Input: part model. Units: mm. Frame: model coordinates. A direction names the side the tool comes from. Give positions to 0.01 mm unless a question says otherwise; leave off trailing zeros. Loops run counter-clockwise (first coordinate to the right, second up) from the corner with the lowest first, then second, coordinate; pieces in that order, holes last.
from build123d import *

# Parameters (mm, degrees)
CROQUIS1_W              = 10
CROQUIS1_H              = 25
SALIENTE_EXTRUIR1_DEPTH = 28
CROQUIS2_R              = 12.5
SALIENTE_EXTRUIR2_DEPTH = 12
REDONDEO1_R             = 5
CORTAR_EXTRUIR1_DEPTH   = 13
CROQUIS5_R              = 9.915
CORTAR_EXTRUIR2_DEPTH   = 7
CROQUIS8_R              = 1.175
CORTAR_EXTRUIR5_DEPTH   = 50.08411164
CROQUIS10_W             = 7
CROQUIS10_H             = 15
SALIENTE_EXTRUIR3_DEPTH = 5
CORTAR_EXTRUIR6_DEPTH   = 7
CORTAR_EXTRUIR7_DEPTH   = 3.85
CHAFL_N1_SIZE           = 4.3
CHAFL_N1_SIZE2          = 5.124540448
REDONDEO2_R             = 1
CORTAR_EXTRUIR8_DEPTH   = 4
REDONDEO3_R             = 3
CROQUIS14_R             = 12.5
CROQUIS14_R_2           = 11.25
SALIENTE_EXTRUIR4_DEPTH = 7.35
CROQUIS15_R             = 12.5
CROQUIS15_R_2           = 11
SALIENTE_EXTRUIR5_DEPTH = 1
CHAFL_N2_SIZE           = 0.5
CHAFL_N3_SIZE           = 0.5
CROQUIS16_R             = 6.5
CORTAR_EXTRUIR9_DEPTH   = 50.43149313


# Some blends are built 0.0001 mm under size
with BuildPart() as part:
    # Croquis1 → Saliente-Extruir1 (new body)
    with BuildSketch(Plane(origin=(0, 0, 0), x_dir=(1, 0, 0), z_dir=(0, 1, 0))):
        with Locations((-5, 12.5)):
            Rectangle(CROQUIS1_W, CROQUIS1_H)
    extrude(amount=SALIENTE_EXTRUIR1_DEPTH)

    # Croquis2 → Saliente-Extruir2 (add)
    with BuildSketch(Plane(origin=(0, 0, 0), x_dir=(0, 0, -1), z_dir=(1, 0, 0))):
        with Locations((12.5, 28)):
            Circle(CROQUIS2_R)
    extrude(amount=-SALIENTE_EXTRUIR2_DEPTH)

    # Croquis3 → Cortar-Revolución1 (revolve, cut)
    with BuildSketch(Plane(origin=(0, 0, 0), x_dir=(0, 0, -1), z_dir=(1, 0, 0))):
        Polygon((21, 0.5), (21, 4), (19, 4), (19, 10), (21, 10), (21, 15), (15.5, 15), (15.5, 41), (12.5, 41), (12.5, 0), (21, 0), align=None)
    revolve(axis=Axis((0, 0, -12.5), (0, 1, 0)), mode=Mode.SUBTRACT)

    # Redondeo1
    redondeo1_edges = [part.edges().sort_by_distance(p)[0] for p in [
        (-5, 0, -25),
        (-5, 0, 0),
    ]]
    fillet(redondeo1_edges, radius=REDONDEO1_R)

    # Croquis4 → Cortar-Extruir1 (cut)
    with BuildSketch(Plane.XZ.offset(-15)):
        Polygon((0, -18.67764788), (5.35, -15.58882394), (5.35, -9.41117606), (0, -6.32235212), (-5.35, -9.41117606), (-5.35, -15.58882394), align=None)
    extrude(amount=-CORTAR_EXTRUIR1_DEPTH, mode=Mode.SUBTRACT)

    # Croquis5 → Cortar-Extruir2 (cut)
    with BuildSketch(Plane(origin=(0, 0, 0), x_dir=(0, 0, -1), z_dir=(1, 0, 0))):
        with Locations((12.5, 28)):
            Circle(CROQUIS5_R)
    extrude(amount=-CORTAR_EXTRUIR2_DEPTH, mode=Mode.SUBTRACT)

    # Croquis8 → Cortar-Extruir5 (cut, through all)
    with BuildSketch(Plane(origin=(0, 0, 0), x_dir=(0, 0, -1), z_dir=(1, 0, 0))):
        with Locations((21.5, 16.5)):
            Circle(CROQUIS8_R)
        with Locations((3.5, 16.5)):
            Circle(CROQUIS8_R)
        with Locations((3.5, 7.5)):
            Circle(CROQUIS8_R)
        with Locations((21.5, 7.5)):
            Circle(CROQUIS8_R)
    extrude(amount=-CORTAR_EXTRUIR5_DEPTH, mode=Mode.SUBTRACT)

    # Croquis10 → Saliente-Extruir3 (add, symmetric)
    with BuildSketch(Plane.XY.offset(-12.5)):
        with Locations((-13.5, 0.5)):
            Rectangle(CROQUIS10_W, CROQUIS10_H)
    extrude(amount=SALIENTE_EXTRUIR3_DEPTH, both=True)

    # Croquis11 → Cortar-Extruir6 (cut)
    with BuildSketch(Plane.XZ.offset(7)):
        with BuildLine():
            Line((-10.743486399, -17.5), (-10, -17.5))
            Line((-10, -17.5), (-10, -7.5))
            Line((-10, -7.5), (-10.743486399, -7.5))
            ThreePointArc((-10.743486399, -7.5), (-11.85, -12.5), (-10.743486399, -17.5))
        make_face()
    extrude(amount=-CORTAR_EXTRUIR6_DEPTH, mode=Mode.SUBTRACT)

    # Croquis12 → Cortar-Extruir7 (cut)
    with BuildSketch(Plane.XZ.offset(7)):
        with BuildLine():
            Line((-13.787722048, -17.5), (-10.743486399, -17.5))
            ThreePointArc((-10.743486399, -17.5), (-11.85, -12.5), (-10.743486399, -7.5))
            Line((-10.743486399, -7.5), (-11.837335004, -7.5))
            ThreePointArc((-11.837335004, -7.5), (-12.358868803, -8.981355103), (-12.6958, -10.515267686))
            Line((-12.6958, -10.515267686), (-13.787722048, -17.5))
        make_face()
    extrude(amount=-CORTAR_EXTRUIR7_DEPTH, mode=Mode.SUBTRACT)

    # Chaflán1
    chafl_n1_edges = [part.edges().sort_by_distance(p)[0] for p in [
        (-17, 8, -12.5),
    ]]
    chafl_n1_side = [part.faces().sort_by_distance(p)[0] for p in [
        (-13.5, 8, -12.5),
    ]]
    chamfer(chafl_n1_edges, length=CHAFL_N1_SIZE, length2=CHAFL_N1_SIZE2, reference=chafl_n1_side[0])

    # Redondeo2
    redondeo2_edges = [part.edges().sort_by_distance(p)[0] for p in [
        (-12.358868803, -3.15, -8.981355103),
        (-13.241761024, -3.15, -14.007633843),
    ]]
    fillet(redondeo2_edges, radius=REDONDEO2_R - 0.0001)  # a hair under: the kernel refuses the full size

    # Croquis13 → Cortar-Extruir8 (cut)
    with BuildSketch(Plane.ZY.offset(10)):
        Polygon((-21.5, 18.830940108), (-23.518653348, 17.665470054), (-23.518653348, 15.334529946), (-21.5, 14.169059892), (-19.481346652, 15.334529946), (-19.481346652, 17.665470054), align=None)
        Polygon((-3.5, 18.830940108), (-5.518653348, 17.665470054), (-5.518653348, 15.334529946), (-3.5, 14.169059892), (-1.481346652, 15.334529946), (-1.481346652, 17.665470054), align=None)
        Polygon((-3.5, 9.830940108), (-5.518653348, 8.665470054), (-5.518653348, 6.334529946), (-3.5, 5.169059892), (-1.481346652, 6.334529946), (-1.481346652, 8.665470054), align=None)
        Polygon((-21.5, 9.830940108), (-23.518653348, 8.665470054), (-23.518653348, 6.334529946), (-21.5, 5.169059892), (-19.481346652, 6.334529946), (-19.481346652, 8.665470054), align=None)
    extrude(amount=-CORTAR_EXTRUIR8_DEPTH, mode=Mode.SUBTRACT)

    # Redondeo3
    redondeo3_edges = [part.edges().sort_by_distance(p)[0] for p in [
        (-17, 2.875459552, -12.5),
        (-12.7, 8, -12.5),
    ]]
    fillet(redondeo3_edges, radius=REDONDEO3_R)

    # Croquis14 → Saliente-Extruir4 (add)
    with BuildSketch(Plane.ZY.offset(12)):
        with Locations((-12.5, 28)):
            Circle(CROQUIS14_R)
        with Locations((-12.5, 28)):
            Circle(CROQUIS14_R_2, mode=Mode.SUBTRACT)
    extrude(amount=SALIENTE_EXTRUIR4_DEPTH)

    # Croquis15 → Saliente-Extruir5 (add)
    with BuildSketch(Plane.ZY.offset(19.35)):
        with Locations((-12.5, 28)):
            Circle(CROQUIS15_R)
        with Locations((-12.5, 28)):
            Circle(CROQUIS15_R_2, mode=Mode.SUBTRACT)
    extrude(amount=SALIENTE_EXTRUIR5_DEPTH)

    # Chaflán2
    chafl_n2_edges = [part.edges().sort_by_distance(p)[0] for p in [
        (-20.35, 28, -23.5),
    ]]
    chamfer(chafl_n2_edges, length=CHAFL_N2_SIZE)

    # Chaflán3
    # the kernel refuses this chamfer: 0.5 mm, written as the material it takes off along each edge
    with BuildSketch(Plane(origin=(-19.35, 28, -12.5), x_dir=(0, 0, 1), z_dir=(0, -1, 0))) as chafl_n3_piece_1_section:
        Polygon((11, CHAFL_N3_SIZE), (11 + CHAFL_N3_SIZE, 0), (11, 0), align=None)
    chafl_n3_piece_1 = revolve(axis=Axis((-19.35, 28, -12.5), (-1, 0, 0)), mode=Mode.PRIVATE)
    chafl_n3_piece_1 = chafl_n3_piece_1 & Plane(origin=(-19.718458847, 28, -12.5), x_dir=(0, 0, 1), z_dir=(1, 0, 0)) * Cylinder(11.25, 46, mode=Mode.PRIVATE)
    add(chafl_n3_piece_1, mode=Mode.SUBTRACT)

    # Croquis16 → Cortar-Extruir9 (cut, through all)
    with BuildSketch(Plane(origin=(-7, 0, 0), x_dir=(0, 0, -1), z_dir=(1, 0, 0))):
        with Locations((12.5, 28)):
            Circle(CROQUIS16_R)
    extrude(amount=-CORTAR_EXTRUIR9_DEPTH, mode=Mode.SUBTRACT)


solid = part.part
(1) Ray query, probe 1 along Z at (x, y) = (-6.25, 17); probe 2 along Y at (x, z) = (-19.5, -12.5); probe 3 along Y at (x, z) = (-9.25, -1.75). Return the intervals inside material, ascending.
Values follow:
probe 1: z = -25 to -23.52, -19.48 to -5.52, -1.48 to 0
probe 2: y = 15.5 to 16.75, 39.25 to 40.5
probe 3: y = 1.2 to 6.18, 8.82 to 15.18, 17.82 to 34.38
(2) Pin query (flat end, axial travel): pin 1 Ø1.2 at (y, z) = (6.5, -21) entering from -X; pin 2 Ø1.5 at (y, z) = (11, -8.5) entering from -X; pin 3 Ø2 at (y, z) = (31, -9) entering from -X; pin 4 Ø1.5 at (x, z) = (-5.5, -3) entering from -Y. Return the tip coordinate at first contact, or that it passes through.
Values follow:
pin 1: stops at x = -6
pin 2: stops at x = -10
pin 3: passes through
pin 4: stops at y = 0.16
(3) Cut plane B-B (y = 7.5). Return the cut outline in (x, z) (3 decimals).
Values follow:
outline: (-12.959, -17.5) - (-10, -17.5) - (-10, -19.481) - (-6, -19.481) - (-6, -20.325) - (0, -20.325) - (0, -19) arc R6.5 cw to (0, -6) - (0, -4.675) - (-6, -4.675) - (-6, -5.519) - (-10, -5.519) - (-10, -7.5) - (-12.959, -7.5) - close; (-10, -25) - (0, -25) - (0, -22.675) - (-6, -22.675) - (-6, -23.519) - (-10, -23.519) - close; (-10, -1.481) - (-6, -1.481) - (-6, -2.325) - (0, -2.325) - (0, 0) - (-10, 0) - close
(4) Mould query, pull axis Z, two halves, no side actions, for faces 1 (the flat face through (-5, 16, 0)), 2 (the flat face through (-11, 8, -12)), 3 (the flat face through (-8, 8, -5.519)). Classes: +Z half, -Z half, draft (parallel to the pull), parting line (faces both ways), or undercut.
Values follow:
face 1: +Z half
face 2: draft
face 3: undercut
(5) Reachability of faces 4 (the flat face through (-14.968, 5.298, -12.43)), 5 (the cylindrical face through (-6.5, 7, -12.6)), 6 (the flat face through (-7, 26, -19)), 7 (the flat face through (-12, -3.15, -16)), 8 (the flat face through (-8.03, 9.24, -2.48)) from +Z, -Z, +X, -X, +Y, -Y: full face, straight path, thin tool, end or side. Return the list, or none.
Values follow:
face 4: +Z, -Z, -X
face 5: +X, -Y
face 6: +X
face 7: -Z, +X, -Y
face 8: -X
(6) Cut plane A-A (x = -1.5). Return the cut outline in (y, z) (3 decimals), and give its area (3 significant figures).
Values follow:
outline: (0.076, -20.867) arc R5 ccw to (5, -25) - (28, -25) arc R12.5 ccw to (40.227, -15.098) - (37.569, -15.098) arc R9.915 cw to (19.628, -17.812) - (15, -17.812) - (15, -20.867) - (10, -20.867) - (10, -18.825) - (4, -18.825) - (4, -20.867) - close; (0.076, -4.133) - (4, -4.133) - (4, -6.175) - (10, -6.175) - (10, -4.133) - (15, -4.133) - (15, -7.188) - (19.628, -7.188) arc R9.915 cw to (37.569, -9.902) - (40.227, -9.902) arc R12.5 ccw to (28, 0) - (5, 0) arc R5 ccw to start; hole circle Ø2.35 at (7.5, -21.5); hole circle Ø2.35 at (7.5, -3.5); hole circle Ø2.35 at (16.5, -21.5); hole circle Ø2.35 at (16.5, -3.5)
area: 330 mm2
(7) Cut plane C-C (y = -1). Return the cut outline in (x, z).
Values follow:
outline: (-17, -17.5) - (-10.74, -17.5) arc R11.85 cw to (-10.74, -7.5) - (-17, -7.5) - close
